```python
from build123d import *

# Parameters (mm, degrees)
SKETCH1_R             = 4.5
BOSS_EXTRUDE1_DEPTH   = 2.5
SKETCH2_W             = 17.5
SKETCH2_H             = 17.5
BOSS_EXTRUDE2_DEPTH   = 300
SKETCH3_W             = 5.2
SKETCH3_H             = 15.2
CUT_EXTRUDE1_DEPTH    = 2.5
F_4_0MM_DOWEL_HOLE1_D = 4
LPATTERN1_COUNT       = 5
LPATTERN1_PITCH       = 60
CHAMFER1_SIZE         = 1


with BuildPart() as part:
    # Sketch1 → Boss-Extrude1 (new, symmetric)
    with BuildSketch(Plane(origin=(0, 0, 0), x_dir=(1, 0, 0), z_dir=(0, 1, 0))):
        with BuildLine():
            Line((-31.821067812, 7.071067812), (-7.071067812, 31.821067812))
            ThreePointArc((-7.071067812, 31.821067812), (0, 34.75), (7.071067812, 31.821067812))
            Line((7.071067812, 31.821067812), (31.821067812, 7.071067812))
            ThreePointArc((31.821067812, 7.071067812), (34.75, 0), (31.821067812, -7.071067812))
            Line((31.821067812, -7.071067812), (7.071067812, -31.821067812))
            ThreePointArc((7.071067812, -31.821067812), (0, -34.75), (-7.071067812, -31.821067812))
            Line((-7.071067812, -31.821067812), (-31.821067812, -7.071067812))
            ThreePointArc((-31.821067812, -7.071067812), (-34.75, 0), (-31.821067812, 7.071067812))
        make_face()
        with Locations(Location((0, 24.75, 0), (0, 0, 270))):
            Circle(SKETCH1_R, mode=Mode.SUBTRACT)
        with Locations(Location((24.75, 0, 0), (0, 0, 270))):
            Circle(SKETCH1_R, mode=Mode.SUBTRACT)
        with Locations(Location((0, -24.75, 0), (0, 0, 270))):
            Circle(SKETCH1_R, mode=Mode.SUBTRACT)
        with Locations(Location((-24.75, 0, 0), (0, 0, 270))):
            Circle(SKETCH1_R, mode=Mode.SUBTRACT)
    extrude(amount=BOSS_EXTRUDE1_DEPTH, both=True)

    # Sketch2 → Boss-Extrude2 (add)
    with BuildSketch(Plane(origin=(0, 2.5, 0), x_dir=(1, 0, 0), z_dir=(0, 1, 0))):
        Rectangle(SKETCH2_W, SKETCH2_H)
    extrude(amount=BOSS_EXTRUDE2_DEPTH)

    # Sketch3 → Cut-Extrude1 (cut)
    with BuildSketch(Plane(origin=(8.75, 0, 0), x_dir=(0, 0, -1), z_dir=(1, 0, 0))):
        with Locations((0, 25.1)):
            Rectangle(SKETCH3_W, SKETCH3_H)
    cut_extrude1 = extrude(amount=-CUT_EXTRUDE1_DEPTH, mode=Mode.SUBTRACT)

    # 4.0mm Dowel Hole1 (through all)
    with Locations(Plane(origin=(6.25, 0, 0), x_dir=(0, 0, -1), z_dir=(1, 0, 0))):
        with Locations((0, 21), (0, 29.2)):
            f_4_0mm_dowel_hole1 = Hole(F_4_0MM_DOWEL_HOLE1_D / 2)

    # LPattern1: Cut-Extrude1, 4.0mm Dowel Hole1 ×5
    with Locations(*[(0, i * LPATTERN1_PITCH, 0) for i in range(1, LPATTERN1_COUNT)]):
        add(cut_extrude1, mode=Mode.SUBTRACT)
        add(f_4_0mm_dowel_hole1, mode=Mode.SUBTRACT)

    # Chamfer1
    chamfer1_edges = [part.edges().sort_by_distance(p)[0] for p in [
        (-8.75, 302.5, 0),
        (0, 302.5, 8.75),
        (8.75, 302.5, 0),
        (0, 302.5, -8.75),
    ]]
    chamfer(chamfer1_edges, length=CHAMFER1_SIZE)


solid = part.part
```
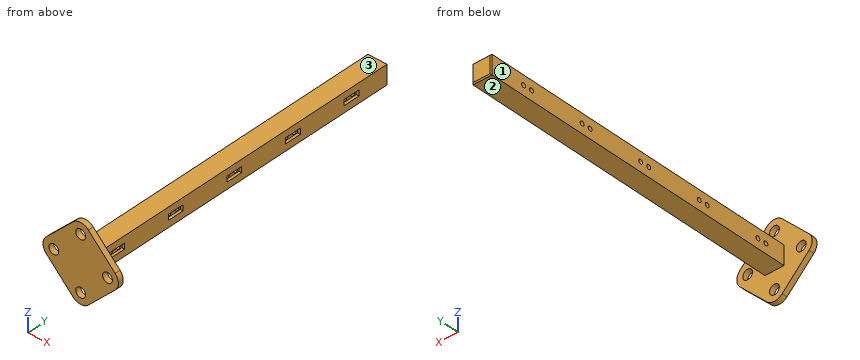
Check sheet for the modelled part. Datum: model origin and axes. Units: mm. Face numbers are marked on the shaded views. A direction names the side the tool comes from. Round coordinates to 2 decimals unless told otherwise and drop trailing zeros. Order: outer loops, then holes, each group sorted by start corner. A loop starts at its lowest first (then second) coordinate and runs counter-clockwise, first axis right, second up.
1) Section check D-D (x = 17.5). Record the boundary of the cut face in (y, z).
2) Tool access check on the marked faces 1, 2 and 3. Record the directions out of +Z, -Z, +X, -X, +Y, -Y that give a thin tool (end or side, any length) a straight path to the whole face; none if there is none.
3) Scan lines: line 1 (X direction, y = 263, z = -7); line 2 (Y direction, x = 18, z = 8). Record each from-to range of solid material in increasing order.
4) Section check C-C (y = 237). Record the boundary of the cut face in (x, z), and give its area (3 significant figures).
5) Go/stop test with flat-tipped pins: pin 1 Ø0.8 at (x, y) = (7.5, 145) entering from +Z; pin 2 Ø12 at (x, z) = (0, -17.5) entering from +Y; pin 3 Ø0.8 at (x, y) = (7, 22.5) entering from -Z. Record where each tip stops, or that it passes through.
6) Section check B-B (x = -24.75). Record the boundary of the cut face in (y, z).
7) Section check A-A (z = -26). Record the boundary of the cut face in (x, y).
Result:
1. outline: (-2.5, -21.39) - (2.5, -21.39) - (2.5, 21.39) - (-2.5, 21.39) - close
2. face 1: +Z, -Z, -X, +Y
2. face 2: -Z, +X, -X, +Y
2. face 3: +Z, +X, -X, +Y
3. line 1: x = -8.75 to 8.75
3. line 2: y = -2.5 to 2.5
4. outline: (-8.75, -8.75) - (8.75, -8.75) - (8.75, 8.75) - (-8.75, 8.75) - close
4. area: 306 mm2
5. pin 1: stops at z = 8.75
5. pin 2: stops at y = 2.5
5. pin 3: stops at z = -8.75
6. outline: (-2.5, -14.14) - (2.5, -14.14) - (2.5, -4.5) - (-2.5, -4.5) - close; (-2.5, 4.5) - (2.5, 4.5) - (2.5, 14.14) - (-2.5, 14.14) - close
7. outline: (-12.89, -2.5) - (-4.32, -2.5) - (-4.32, 2.5) - (-12.89, 2.5) - close; (4.32, -2.5) - (12.89, -2.5) - (12.89, 2.5) - (4.32, 2.5) - close
